Verification items for the finished model (mm, model axes). A direction names the side the tool comes from. Round coordinates to 2 decimals unless told otherwise and drop trailing zeros. Order: outer loops, then holes, each group sorted by start corner. A loop starts at its lowest first (then second) coordinate and runs counter-clockwise, first axis right, second up. Notation, with made-up numbers: (50, -32.5) -> (54, -32.5) arc R30 cw to (54, 6.5) -> close; hole circle Ø8 at (83, -22.5). An arc over 180 degrees is marked (long way). Put each result on its own line as item: value.
from build123d import *

# Parameters (mm, degrees)
ESQUISSE1_W                  = 13
ESQUISSE1_H                  = 29
ESQUISSE2_R                  = 11.5
ENL_V_MAT_EXTRU_1_DEPTH      = 4
CHANFREIN1_SIZE              = 1
ESQUISSE4_R                  = 8
ENL_V_MAT_EXTRU_2_DEPTH      = 10
ENL_V_MAT_EXTRU_4_DEPTH      = 35.336569502
ENL_V_MAT_EXTRU_4_DEPTH_BACK = 35.336569502
ESQUISSE6_R                  = 5
ENL_V_MAT_EXTRU_5_REACH      = 42.559
ESQUISSE8_R                  = 3


with BuildPart() as part:
    # Esquisse1 → Base-Révolution (revolve)
    with BuildSketch(Plane.XY, mode=Mode.PRIVATE) as base_r_volution_sk:
        with Locations((6.5, 14.5)):
            Rectangle(ESQUISSE1_W, ESQUISSE1_H)
    revolve(base_r_volution_sk.sketch.rotate(Axis((0, 0, 0), (0, 1, 0)), 90), axis=Axis((0, 0, 0), (0, 1, 0)))

    # Esquisse2 → Enlèv. mat.-Extru.1 (cut)
    with BuildSketch(Plane.XZ):
        with Locations(Location((0, 0, 0), (0, 0, 270))):
            Circle(ESQUISSE2_R)
    extrude(amount=-ENL_V_MAT_EXTRU_1_DEPTH, mode=Mode.SUBTRACT)

    # Chanfrein1
    chanfrein1_edges = [part.edges().sort_by_distance(p)[0] for p in [
        (0, 0, 13),
        (0, 29, 13),
    ]]
    chamfer(chanfrein1_edges, length=CHANFREIN1_SIZE)

    # Esquisse3 → Enlèvement de matière-Révolution1 (revolve, cut)
    with BuildSketch(Plane(origin=(0, 0, 0), x_dir=(1, 0, 0), z_dir=(0, 1, 0))):
        Polygon((0, 12.2), (16.5, 12.2), (21.5, 17.2), (0, 17.2), align=None)
    revolve(axis=Axis((0, 0, 0), (0, 0, -1)), mode=Mode.SUBTRACT)

    # Esquisse4 → Enlèv. mat.-Extru.2 (cut)
    with BuildSketch(Plane.XZ.offset(-4)):
        with Locations(Location((0, 0, 0), (0, 0, 270))):
            Circle(ESQUISSE4_R)
    extrude(amount=-ENL_V_MAT_EXTRU_2_DEPTH, mode=Mode.SUBTRACT)

    # Esquisse6 → Enlèv. mat.-Extru.4 (cut, two sides: drawn at the far end of the back side and taken through both)
    with BuildSketch(Plane(origin=(0, 0, 0), x_dir=(0, 0, -1), z_dir=(1, 0, 0)).offset(-ENL_V_MAT_EXTRU_4_DEPTH_BACK)):
        with Locations((0, 20.2)):
            Circle(ESQUISSE6_R)
    extrude(amount=ENL_V_MAT_EXTRU_4_DEPTH + ENL_V_MAT_EXTRU_4_DEPTH_BACK, mode=Mode.SUBTRACT)

    # Esquisse7 → Enlèvement de matière-Révolution2 (revolve, cut)
    with BuildSketch(Plane(origin=(0, 29, 0), x_dir=(-1, 0, 0), z_dir=(0, 1, 0))):
        Polygon((-11.25, 0), (-11.25, 17.5), (-16.25, 22.5), (-16.25, 0), align=None)
        Polygon((11.25, 0), (11.25, 17.5), (16.25, 22.5), (16.25, 0), align=None)
    revolve(axis=Axis((0, 29, 0), (1, 0, 0)), mode=Mode.SUBTRACT)

    # Esquisse8 → Enlèv. mat.-Extru.5 (cut, up to next)
    with BuildSketch(Plane(origin=(0, 0, -12.2), x_dir=(-1, 0, 0), z_dir=(0, 0, -1)), mode=Mode.PRIVATE) as enl_v_mat_extru_5_sk1:
        with Locations((0, 8)):
            Circle(ESQUISSE8_R)
    enl_v_mat_extru_5_tool1 = extrude(enl_v_mat_extru_5_sk1.sketch, amount=-ENL_V_MAT_EXTRU_5_REACH, mode=Mode.PRIVATE) & part.part
    add(enl_v_mat_extru_5_tool1.solids().sort_by_distance((0, 8, -12.2))[0], mode=Mode.SUBTRACT)


solid = part.part
Item 1: Release check for a two-part mould opening along X. For faces 1 (the flat face through (11.25, 26, 0)), 2 (the cylindrical face through (3, 8, -10)), 3 (the cylindrical face through (-4.868, 8.93, 6.349)), 4 (the conical face through (-11.75, 11, 0.1)) record: +X half, -X half, draft (parallel to the pull), parting line (faces both ways), or undercut.
Check sheet entries:
face 1: +X half
face 2: undercut
face 3: undercut
face 4: -X half
Item 2: Gauge pin test, flat ends, axial feed: pin 1 Ø1 at (x, y) = (-7, 3) entering from +Z; pin 2 Ø13 at (x, z) = (0, 0) entering from -Y; pin 3 Ø2.5 at (x, y) = (2, 4.5) entering from -Z. Record the tip position at first contact, or that the pin passes through.
Check sheet entries:
pin 1: stops at z = 11.26
pin 2: stops at y = 14
pin 3: stops at z = -12.2
Item 3: Material ranges on L1, parallel to Y at x = 0, z = -10.1; L2, parallel to X at y = 2.95, z = 0; L3, parallel to X at y = 7, z = 0, recorded low to high. Write a range as [from, to].
Check sheet entries:
L1: y = [4, 5], [11, 29]
L2: x = [-13, -11.5], [11.5, 13]
L3: x = [-13, -8], [8, 13]
Item 4: Section check C-C on y = 20.2. Record the boundary of the cut face in (x, z), then the cut area to 3 significant figures.
Check sheet entries:
outline: (-11.25, -6.51) arc R13 ccw to (11.25, -6.51) -> (11.25, -5) -> (-11.25, -5) -> close; (-11.25, 5) -> (11.25, 5) -> (11.25, 6.51) arc R13 ccw to (-11.25, 6.51) -> close
area: 275 mm^2
Item 5: Tool access check on faces 5 (the cylindrical face through (9.7, 1.97, -6.18)), 6 (the flat face through (10, 0, 6)), 7 (the flat face through (-11.25, 26, 0)). Record the directions out of +Z, -Z, +X, -X, +Y, -Y that give a thin tool (end or side, any length) a straight path to the whole face; none if there is none.
Check sheet entries:
face 5: -Y
face 6: +Z, -Z, +X, -X, -Y
face 7: -X, +Y
Item 6: Section check B-B on z = 0. Record the boundary of the cut face in (x, y).
Check sheet entries:
outline: (-13, 1) -> (-12, 0) -> (-11.5, 0) -> (-11.5, 4) -> (-8, 4) -> (-8, 14) -> (8, 14) -> (8, 4) -> (11.5, 4) -> (11.5, 0) -> (12, 0) -> (13, 1) -> (13, 9.75) -> (11.25, 11.5) -> (11.25, 15.2) -> (-11.25, 15.2) -> (-11.25, 11.5) -> (-13, 9.75) -> close; (-11.25, 25.2) -> (11.25, 25.2) -> (11.25, 29) -> (-11.25, 29) -> close
Item 7: Section check A-A on x = 0. Record the boundary of the cut face in (y, z), then the cut area to 3 significant figures.
Check sheet entries:
outline: (0, -12) -> (0.2, -12.2) -> (5, -12.2) -> (5, -8) -> (4, -8) -> (4, -11.5) -> (0, -11.5) -> close; (0, 11.5) -> (4, 11.5) -> (4, 8) -> (14, 8) -> (14, -8) -> (11, -8) -> (11, -12.2) -> (16.5, -12.2) -> (17.3, -13) -> (28, -13) -> (29, -12) -> (29, 12) -> (28, 13) -> (1, 13) -> (0, 12) -> close; hole circle Ø10 at (20.2, 0)
area: 383 mm^2
